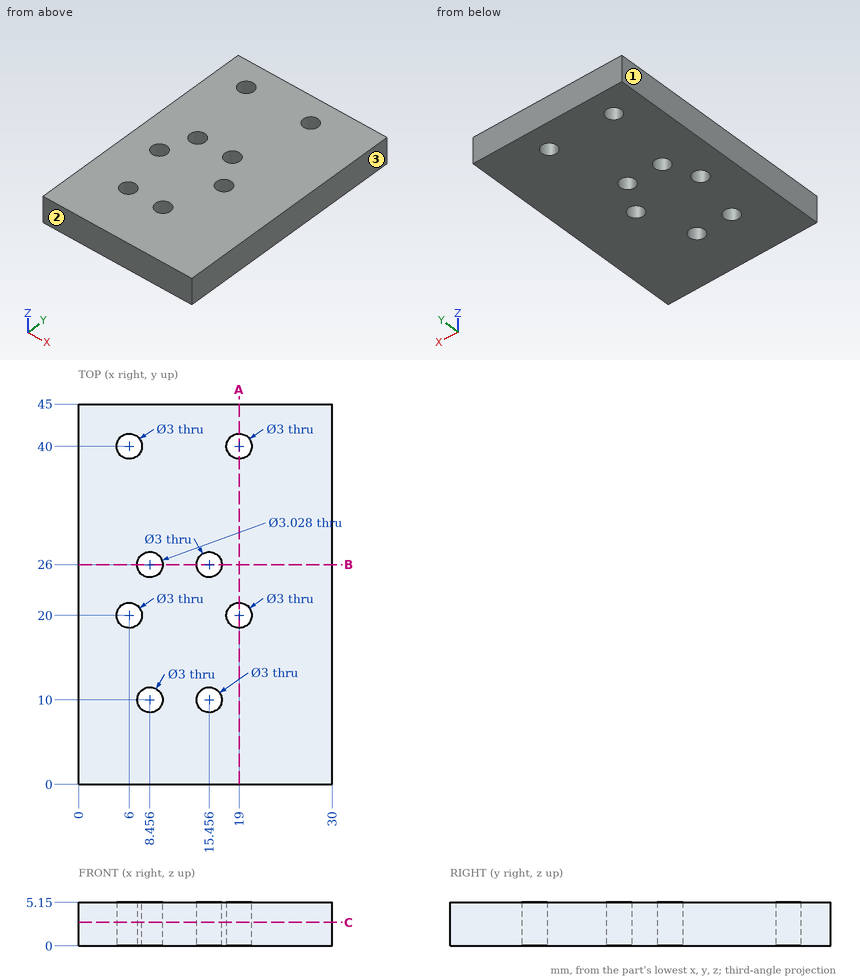
Drawing for the job (mm, zero at the part's lowest x, y, z). Coordinates: 2 decimals unless noted, no trailing zeros. Loops run counter-clockwise (first coordinate to the right, second up) from the corner with the lowest first, then second, coordinate; pieces in that order, holes last. Notation, with made-up numbers: (71.25, 14.5) - (113.25, 14.5) arc R6 ccw to (113.25, 19.5) - close; hole circle Ø4 at (19.5, 88.5). An arc over 180 degrees is marked (long way). Return JSON: item names as keys, results as strings.
1. Mould opens along X. For the marked faces 1, 2 and 3 say: released by +X, released by -X, zero draft, split by the parting line, or undercut.
Result:
{"face 1": "released by -X", "face 2": "zero draft", "face 3": "released by +X"}
2. Band-saw the part on C-C (z = 2.8). State how many separate pieces and enclosed holes the cut face has, and give its area (3 significant figures).
Result:
{"separate pieces": "1", "enclosed holes": "8", "area": "1,290 mm2"}
3. Band-saw the part on A-A (x = 19). Give the cut face in (y, z), and give its area (3 significant figures).
Result:
{"outline": "(0, 0) - (18.5, 0) - (18.5, 5.15) - (0, 5.15) - close; (21.5, 0) - (38.5, 0) - (38.5, 5.15) - (21.5, 5.15) - close; (41.5, 0) - (45, 0) - (45, 5.15) - (41.5, 5.15) - close", "area": "201 mm2"}
4. Probe L1, parallel to X at y = 10, z = 3.5; L2, parallel to X at y = 20, z = 1.4; L3, parallel to Y at x = 9, z = 2.85. List the from-to ranges inside material, lowest first. Write a range as from..to.
Result:
{"L1": "x = 0..6.96, 9.96..13.96, 16.96..30", "L2": "x = 0..4.5, 7.5..17.5, 20.5..30", "L3": "y = 0..8.6, 11.4..24.59, 27.41..45"}
5. Drop flat-ended pins along their axis: pin 1 (1.8 mm diameter, centred on x = 8.46, y = 26, fed in from -Z); pin 2 (1.5 mm diameter, centred on x = 26.5, y = 21, fed in from -Z). Give the stop position or say it passes through.
Result:
{"pin 1": "passes through", "pin 2": "stops at z = 0"}
6. Band-saw the part on B-B (y = 26). Give the cut face in (x, z).
Result:
{"outline": "(0, 0) - (6.94, 0) - (6.94, 5.15) - (0, 5.15) - close; (9.97, 0) - (13.96, 0) - (13.96, 5.15) - (9.97, 5.15) - close; (16.96, 0) - (30, 0) - (30, 5.15) - (16.96, 5.15) - close"}
